CAD build for the part. Positions are in the model's coordinates, mm. Round coordinates to 2 decimals unless told otherwise and drop trailing zeros. Use a Markdown table: item, result. Add a question column.
(1) Band-saw the part on C-C, the plane x = 18. Give the number of separate pieces and of enclosed holes in the cut face, and give its area (3 significant figures).
(2) Wall check: L1, parallel to X at y = 19, z = 0.3; L2, parallel to Y at x = 18, z = 0.7; L3, parallel to X at y = 14, z = 1.15. Give the ranges that are in metal, low to high.
(3) Flat gauge pin, fed straight in: P1, Ø1, axis at x = 94.5, z = 1, coming from the -Y side. Where does the tip first touch, or does it go through?
(4) Two-plate mould, pull along Y, no slides. Class faces 1 (the face through (81, 39, 2)), 2 (the face through (18, 34, 1)): released by +Y, released by -Y, zero draft, split by the parting line, or undercut.
from build123d import *

# Parameters (mm, degrees)
SKICA1_W                 = 160
SKICA1_H                 = 46
SKICA1_R                 = 2
P_IDAT_VYSUNUT_M1_DEPTH  = 2
SKICA2_W                 = 166
SKICA2_H                 = 52
SKICA2_W_2               = 160
SKICA2_H_2               = 46
P_IDAT_VYSUNUT_M4_DEPTH  = 2
SKICA3_W                 = 63
SKICA3_H                 = 32
ODEBRAT_VYSUNUT_M1_DEPTH = 171.217507913
SKICA4_W                 = 16.5
SKICA4_H                 = 7.5
ODEBRAT_VYSUNUT_M2_DEPTH = 171.217507913
ZAOBLIT14_R              = 2
SKICA5_R                 = 2
ODEBRAT_VYSUNUT_M3_DEPTH = 171.217507913
ZAOBLIT16_R              = 2


with BuildPart() as part:
    # Skica1 → Přidat vysunutím1 (new body)
    with BuildSketch(Plane.XY):
        with Locations((80, 23)):
            Rectangle(SKICA1_W, SKICA1_H)
        with Locations((7.6, 25)):
            Circle(SKICA1_R, mode=Mode.SUBTRACT)
        with Locations((8.3, 9.7)):
            Circle(SKICA1_R, mode=Mode.SUBTRACT)
        with Locations((142.7, 26.2)):
            Circle(SKICA1_R, mode=Mode.SUBTRACT)
        with Locations((142.7, 8.4)):
            Circle(SKICA1_R, mode=Mode.SUBTRACT)
    extrude(amount=P_IDAT_VYSUNUT_M1_DEPTH)

    # Skica2 → Přidat vysunutím4 (add)
    with BuildSketch(Plane(origin=(0, 0, 0), x_dir=(-1, 0, 0), z_dir=(0, 0, -1))):
        with Locations((-80, 23)):
            Rectangle(SKICA2_W, SKICA2_H)
        with Locations((-80, 23)):
            Rectangle(SKICA2_W_2, SKICA2_H_2, mode=Mode.SUBTRACT)
    extrude(amount=-P_IDAT_VYSUNUT_M4_DEPTH)

    # Skica3 → Odebrat vysunutím1 (cut, through all)
    with BuildSketch(Plane.XY.offset(2)):
        with Locations((94.5, 17)):
            Rectangle(SKICA3_W, SKICA3_H)
    extrude(amount=-ODEBRAT_VYSUNUT_M1_DEPTH, mode=Mode.SUBTRACT)

    # Skica4 → Odebrat vysunutím2 (cut, through all)
    with BuildSketch(Plane.XY.offset(2)):
        with Locations((96.75, 39.75)):
            Rectangle(SKICA4_W, SKICA4_H)
    extrude(amount=-ODEBRAT_VYSUNUT_M2_DEPTH, mode=Mode.SUBTRACT)

    # Zaoblit14
    zaoblit14_edges = [part.edges().sort_by_distance(p)[0] for p in [
        (-3, 23, 2),
        (80, 49, 2),
        (80, -3, 2),
        (163, 23, 2),
    ]]
    fillet(zaoblit14_edges, radius=ZAOBLIT14_R - 0.0001)  # a hair under: the kernel refuses the full size

    # Skica5 → Odebrat vysunutím3 (cut, through all)
    with BuildSketch(Plane.XY.offset(2)):
        with Locations((18, 15)):
            Circle(SKICA5_R)
        with Locations((18, 26)):
            Circle(SKICA5_R)
        with Locations((18, 36)):
            Circle(SKICA5_R)
    extrude(amount=-ODEBRAT_VYSUNUT_M3_DEPTH, mode=Mode.SUBTRACT)

    # Zaoblit16
    zaoblit16_edges = [part.edges().sort_by_distance(p)[0] for p in [
        (94.5, 1, 2),
        (126, 17, 2),
        (94.5, 33, 2),
        (63, 17, 2),
    ]]
    fillet(zaoblit16_edges, radius=ZAOBLIT16_R - 0.0001)  # a hair under: the kernel refuses the full size


solid = part.part
Return value:
| question | item | result |
|---|---|---|
| 1 | separate pieces | 4 |
| 1 | enclosed holes | 0 |
| 1 | area | 78.3 mm^2 |
| 2 | L1 | -2.98 to 62.98, 126.02 to 162.98 |
| 2 | L2 | -2.87 to 13, 17 to 24, 28 to 34, 38 to 48.87 |
| 2 | L3 | -2.64 to 16.27, 19.73 to 62.64, 126.36 to 162.64 |
| 3 | P1 | y = -2.94 |
| 4 | face 1 | zero draft |
| 4 | face 2 | undercut |
